Work out the finished part from the listing and answer in its coordinate system (mm). A direction names the side the tool comes from. Give positions to 0.01 mm unless a question says otherwise; leave off trailing zeros. Loops run counter-clockwise (first coordinate to the right, second up) from the corner with the lowest first, then second, coordinate; pieces in that order, holes last. Notation, with made-up numbers: M 88,82.25 L 141,82.25 A22 ccw 141,92.25 Z; hole C 54,6.25 d1. An arc over 180 degrees is marked long. Write item = value, one per line. Start each with the question number.
1. Section A-A on x = 0 is taken. Determine the outline of the cut face in (y, z) (3 decimals).
2. The mould has two halves that part along Z. Classify faces 1 (the face through (1, 0, -1)), 2 (the face through (-7.493, -21.232, 0.33)), 3 (the face through (-1.873, -20.527, 0.082)): released by +Z, released by -Z, zero draft, split by the parting line, or undercut.
3. Section C-C on y = -11 is taken. Determine the outline of the cut face in (x, z) (3 decimals).
4. Section B-B on z = 0 is taken. Determine the outline of the cut face in (x, y) (3 decimals), plus the area to 3 significant figures.
5. For faces 4 (the face through (1, -20, 6)), 5 (the face through (1, -22.5, 6)), 6 (the face through (0.27, -4.68, -1.22)), determine the directions among +Z, -Z, +X, -X, +Y, -Y from which every point of the face is accessible in a straight line to the end or side of a thin tool.
6. Consider L1, parallel to Z at x = 0, y = -5 (3 decimals); L2, parallel to Y at x = 2.5, z = 6.5; L3, parallel to Z at x = 0, y = -18.5 (3 decimals). Determine where each line is inside the solid, lowest interval first. Write a range as [from, to].
7. Section D-D on x = 3.5 is taken. Determine the outline of the cut face in (y, z).
8. Flat-ended cylindrical pins translate along their axes: pin 1 Ø1.5 at (x, z) = (0, 0) entering from -Y; pin 2 Ø2 at (x, z) = (4.5, -6) entering from -Y; pin 3 Ø8 at (x, y) = (-4.5, -12) entering from -Z; pin 4 Ø1 at (x, y) = (-5, -26) entering from -Z (3 decimals). Find the tip coordinate at first contact, or state that the pin passes through.
```python
from build123d import *

# Parameters (mm, degrees)
F0_R           = 5.625
F1_DEPTH       = 31.25
F3_R           = 7.5
F4_DEPTH       = 2.5
F6_D           = 2.5
F6_DEPTH       = 40
F6_CBORE_D     = 3.75
F6_CBORE_DEPTH = 21.75


with BuildPart() as f1:
    # F0 (on Front) → F1 (new body)
    with BuildSketch(Plane.XZ):
        Circle(F0_R)
    extrude(amount=F1_DEPTH)

    # F3 (on offset) → F4 (join)
    with BuildSketch(Plane.XZ.offset(20)):
        Circle(F3_R)
    extrude(amount=F4_DEPTH)

    # F6
    with Locations(Plane.XZ.offset(31.25)):
        with Locations((0, 0)):
            CounterBoreHole(F6_D / 2, F6_CBORE_D / 2, F6_CBORE_DEPTH, depth=F6_DEPTH)


solid = f1.part
```
Verdict:
q1.outline = M -31.25,-5.625 L -22.5,-5.625 L -22.5,-7.5 L -20,-7.5 L -20,-5.625 L 0,-5.625 L 0,-1.25 L -9.5,-1.25 L -9.5,-1.875 L -31.25,-1.875 Z; M -31.25,1.875 L -9.5,1.875 L -9.5,1.25 L 0,1.25 L 0,5.625 L -20,5.625 L -20,7.5 L -22.5,7.5 L -22.5,5.625 L -31.25,5.625 Z
q2.face_1 = zero draft
q2.face_2 = split by the parting line
q2.face_3 = undercut
q3.outline = C 0,0 d11.25; hole C 0,0 d3.75
q4.outline = M -7.5,-22.5 L -5.625,-22.5 L -5.625,-31.25 L -1.875,-31.25 L -1.875,-9.5 L -1.25,-9.5 L -1.25,0 L -5.625,0 L -5.625,-20 L -7.5,-20 Z; M 1.25,-9.5 L 1.875,-9.5 L 1.875,-31.25 L 5.625,-31.25 L 5.625,-22.5 L 7.5,-22.5 L 7.5,-20 L 5.625,-20 L 5.625,0 L 1.25,0 Z
q4.area = 256 mm2
q5.face_4 = +Y
q5.face_5 = -Y
q5.face_6 = +Y, -Y
q6.L1 = [-5.625, -1.25], [1.25, 5.625]
q6.L2 = [-22.5, -20]
q6.L3 = [-5.625, -1.875], [1.875, 5.625]
q7.outline = M -31.25,-4.4 L -22.5,-4.4 L -22.5,-6.63 L -20,-6.63 L -20,-4.4 L 0,-4.4 L 0,4.4 L -20,4.4 L -20,6.63 L -22.5,6.63 L -22.5,4.4 L -31.25,4.4 Z
q8.pin_1 = through
q8.pin_2 = -22.5
q8.pin_3 = -5.6
q8.pin_4 = -3.375
